Work out the finished part from the listing and answer in its coordinate system (mm). Face numbers are marked on the shaded views. A direction names the side the tool comes from. Round coordinates to 2 decimals unless told otherwise and drop trailing zeros. Write each loop counter-clockwise with the first axis right and the second up, starting at its lowest first coordinate (ties: lowest second). Pieces come first, ordered by that corner, then holes. Notation, with made-up numbers: M 1,68.25 L 34,68.25 A13 ccw 34,93.25 Z; hole C 61,53.5 d3. An arc over 180 degrees is marked long. Answer in a Markdown table with one row per item.
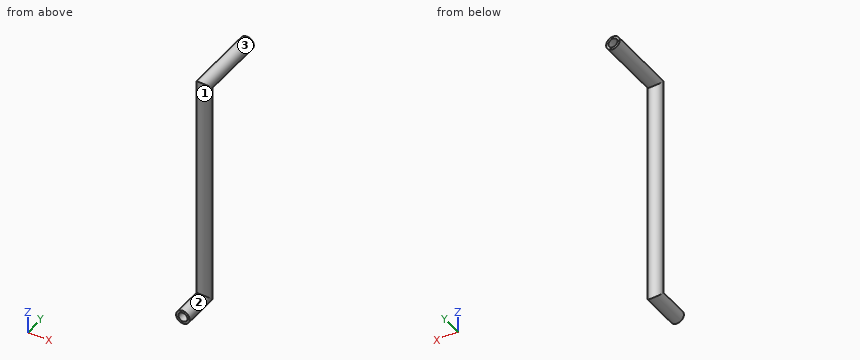
```python
from build123d import *

# Parameters (mm, degrees)
SKETCH4_R   = 60
SKETCH4_R_2 = 40


with BuildPart() as part:
    # Sweep1: sweep along a path in Sketch1
    with BuildLine(Plane(origin=(0, 0, 0), x_dir=(0, 0, -1), z_dir=(1, 0, 0))) as sweep1_path:
        Line((0, 0), (0, 300))
        Line((0, 300), (-2000, 300))
        Line((-2000, 300), (-2000, 900))
    # Sketch4 → Sweep1 (sweep)
    with BuildSketch(Plane(origin=(0, 0, 0), x_dir=(1, 0, 0), z_dir=(0, 1, 0))):
        Circle(SKETCH4_R)
        Circle(SKETCH4_R_2, mode=Mode.SUBTRACT)
    sweep(path=sweep1_path.line, transition=Transition.RIGHT)


solid = part.part
```
1. The part is cut by section C-C (z = 0). Determine the outline of the cut face in (x, y), plus the area to 3 significant figures.
Calculated:
| item | result |
|---|---|
| outline | M -60,0 L -40,0 L -40,300 A40 cw 40,300 L 40,0 L 60,0 L 60,300 A60 ccw -60,300 Z |
| area | 15,100 mm² |
2. Consider line 1 along Z through (x, y) = (-4.5, 59); line 2 along X through (y, z) = (233, 0); line 3 along Y through (x, z) = (0, 572.5). Determine where each line is inside the solid, lowest interval first. Write a range as from..to.
Calculated:
| item | result |
|---|---|
| line 1 | z = -59.83..-39.75, 39.75..59.83 |
| line 2 | x = -60..-40, 40..60 |
| line 3 | y = 240..260, 340..360 |
3. The part is cut by section D-D (z = 1017). Determine the outline of the cut face in (x, y), plus the area to 3 significant figures.
Calculated:
| item | result |
|---|---|
| outline | C 0,300 d120; hole C 0,300 d80 |
| area | 6,280 mm² |
4. The part is cut by section A-A (y = 300). Determine the outline of the cut face in (x, z).
Calculated:
| item | result |
|---|---|
| outline | M -60,0 A60 ccw 60,0 L 60,2000 A60 ccw -60,2000 Z; hole M -40,0 A40 ccw 40,0 L 40,2000 A40 ccw -40,2000 Z |
5. The part is cut by section B-B (x = 0). Determine the outline of the cut face in (y, z).
Calculated:
| item | result |
|---|---|
| outline | M 0,-60 L 360,-60 L 360,1940 L 900,1940 L 900,1960 L 340,1960 L 340,-40 L 0,-40 Z; M 0,40 L 260,40 L 260,2040 L 900,2040 L 900,2060 L 240,2060 L 240,60 L 0,60 Z |
6. A tool of negligible diameter and unlimited length cuts with its end or side. For the marked faces 1, 2 and 3, from which of +Z, -Z, +X, -X, +Y, -Y can it reach the whole face along a straight path? Write none if from no direction.
Calculated:
| item | result |
|---|---|
| face 1 | none |
| face 2 | -Y |
| face 3 | +Y |
7. Given pin 1 (12 mm diameter, centred on x = -7, y = 364, fed in from -Z); pin 2 (4 mm diameter, centred on x = -36, y = 107.5, fed in from +Z); pin 3 (3 mm diameter, centred on x = -14.5, z = 402.5, fed in from +Y), each flat-ended and moving along its own axis, determine where each tip first touches the part or whether it passes through.
Calculated:
| item | result |
|---|---|
| pin 1 | stops at z = -59.94 |
| pin 2 | stops at z = 49.44 |
| pin 3 | stops at y = 358.57 |
